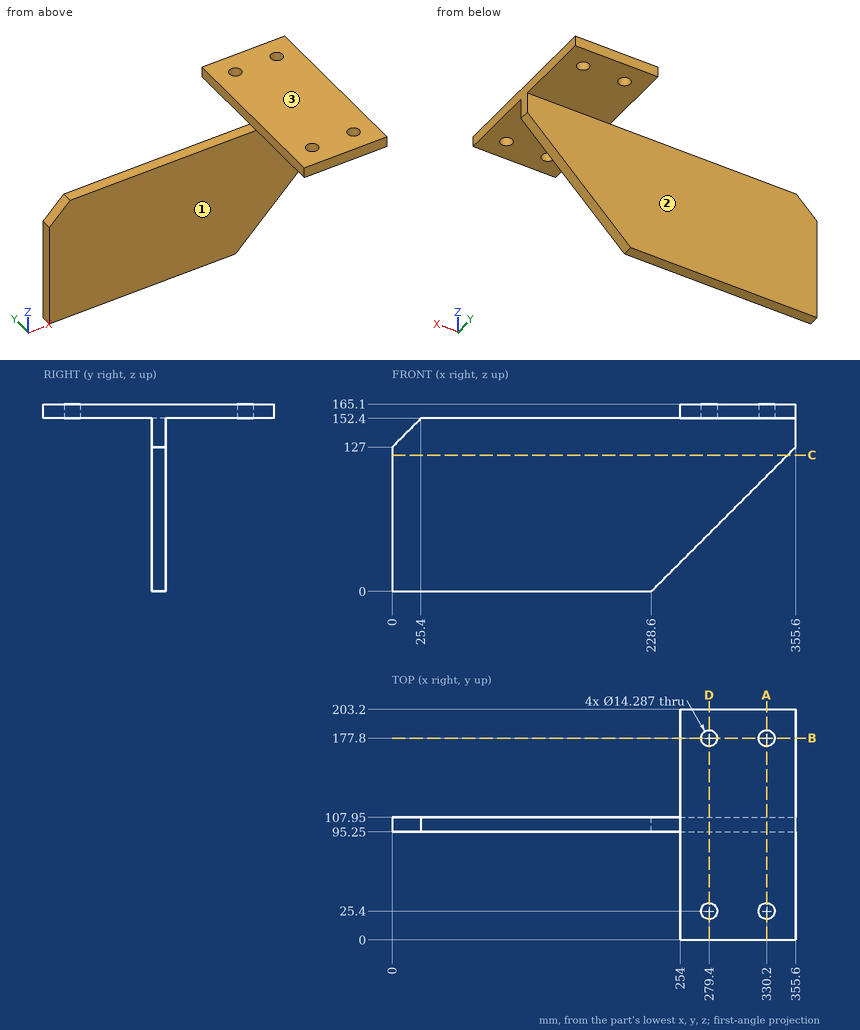
Study the drawing (mm; zero at the part's minimum x, y, z) and answer. A direction names the side the tool comes from. Give positions to 0.01 mm unless a question says otherwise; leave off trailing zeros. Write each loop counter-clockwise with the first axis right and the second up, starting at its lowest first coordinate (ties: lowest second). Pieces come first, ordered by that corner, then holes. Notation, with made-up numbers: (-22, 72.25) -> (35, 72.25) arc R21 cw to (35, 91.25) -> close; hole circle Ø9 at (-22.75, 53). An arc over 180 degrees is marked (long way). Write item = value, one per line. Start each with the question number.
1) Each of these flat-tipped pins is pushed along its axis until it touches: pin 1 (12 mm diameter, centred on x = 280.5, y = 168, fed in from -Z); pin 2 (1 mm diameter, centred on x = 37, z = 59.5, fed in from +Y); pin 3 (8 mm diameter, centred on x = 159.5, z = 51.5, fed in from -Y). Where does it stop, or does it pass through?
2) The part is cut by section C-C, the plane z = 120. Determine the outline of the cut face in (x, y).
3) Straight lines are drawn through the part: line 1 along X through (y, z) = (177, 158); line 2 along Y through (x, z) = (330.2, 157.75); line 3 along Z through (x, y) = (266, 89.5). For each, find the intervals that lie inside material, in ascending order.
4) The part is cut by section A-A, the plane x = 330.2. Determine the outline of the cut face in (y, z), and give its area (3 significant figures).
5) The part is cut by section D-D, the plane x = 279.4. Determine the outline of the cut face in (y, z), and give its area (3 significant figures).
6) The part is cut by section B-B, the plane y = 177.8. Determine the outline of the cut face in (x, z).
7) Which of the six approach directions +Z, -Z, +X, -X, +Y, -Y give full straight-line access (tool end or side, diameter ignored) to the marked faces 1, 2 and 3?
Solutions:
q1.pin_1 = 152.4
q1.pin_2 = 107.95
q1.pin_3 = 95.25
q2.outline = (0, 95.25) -> (348.6, 95.25) -> (348.6, 107.95) -> (0, 107.95) -> close
q3.line_1 = 254 to 272.3, 286.5 to 323.1, 337.3 to 355.6
q3.line_2 = 0 to 18.26, 32.54 to 170.66, 184.94 to 203.2
q3.line_3 = 152.4 to 165.1
q4.outline = (0, 152.4) -> (18.26, 152.4) -> (18.26, 165.1) -> (0, 165.1) -> close; (32.54, 152.4) -> (95.25, 152.4) -> (95.25, 101.6) -> (107.95, 101.6) -> (107.95, 152.4) -> (170.66, 152.4) -> (170.66, 165.1) -> (32.54, 165.1) -> close; (184.94, 152.4) -> (203.2, 152.4) -> (203.2, 165.1) -> (184.94, 165.1) -> close
q4.area = 2,860 mm²
q5.outline = (0, 152.4) -> (18.26, 152.4) -> (18.26, 165.1) -> (0, 165.1) -> close; (32.54, 152.4) -> (95.25, 152.4) -> (95.25, 50.8) -> (107.95, 50.8) -> (107.95, 152.4) -> (170.66, 152.4) -> (170.66, 165.1) -> (32.54, 165.1) -> close; (184.94, 152.4) -> (203.2, 152.4) -> (203.2, 165.1) -> (184.94, 165.1) -> close
q5.area = 3,510 mm²
q6.outline = (254, 152.4) -> (272.26, 152.4) -> (272.26, 165.1) -> (254, 165.1) -> close; (286.54, 152.4) -> (323.06, 152.4) -> (323.06, 165.1) -> (286.54, 165.1) -> close; (337.34, 152.4) -> (355.6, 152.4) -> (355.6, 165.1) -> (337.34, 165.1) -> close
q7.face_1 = -Z, +X, -X, -Y
q7.face_2 = -Z, +X, -X, +Y
q7.face_3 = +Z, +X, -X, +Y, -Y
